from build123d import *

# Parameters (mm, degrees)
SKETCH1_R               = 225
BOSS_EXTRUDE1_DEPTH     = 30
SKETCH2_R               = 210
CUT_EXTRUDE1_DEPTH      = 1
CUT_EXTRUDE1_DEPTH_BACK = 31
SKETCH3_W               = 50
SKETCH3_H               = 20
BOSS_EXTRUDE2_DEPTH     = 50
SKETCH4_W               = 50
SKETCH4_H               = 20.506281323
BOSS_EXTRUDE3_DEPTH     = 110
SKETCH5_W               = 50
SKETCH5_H               = 25
BOSS_EXTRUDE7_DEPTH     = 40
SKETCH6_W               = 27.39243627
SKETCH6_H               = 13.13
BOSS_EXTRUDE8_DEPTH     = 15
SKETCH7_R               = 1.25
BOSS_EXTRUDE9_DEPTH     = 10
SKETCH8_R               = 1.25
BOSS_EXTRUDE10_DEPTH    = 10
FILLET14_R              = 3
FILLET15_R              = 2.5
FILLET17_R              = 3


with BuildPart() as part:
    # Sketch1 → Boss-Extrude1 (new body)
    with BuildSketch(Plane(origin=(0, 0, 0), x_dir=(1, 0, 0), z_dir=(0, 1, 0))):
        Circle(SKETCH1_R)
    extrude(amount=BOSS_EXTRUDE1_DEPTH)

    # Sketch2 → Cut-Extrude1 (cut, two sides)
    with BuildSketch(Plane(origin=(0, 30, 0), x_dir=(1, 0, 0), z_dir=(0, 1, 0))) as cut_extrude1_sk:
        Circle(SKETCH2_R)
    extrude(amount=CUT_EXTRUDE1_DEPTH, mode=Mode.SUBTRACT)
    extrude(cut_extrude1_sk.sketch, amount=-CUT_EXTRUDE1_DEPTH_BACK, mode=Mode.SUBTRACT)

    # Sketch3 → Boss-Extrude2 (add)
    with BuildSketch(Plane.XY.offset(-214.619360396)):
        with Locations((0, 15)):
            Rectangle(SKETCH3_W, SKETCH3_H)
    extrude(amount=-BOSS_EXTRUDE2_DEPTH)

    # Sketch4 → Boss-Extrude3 (add)
    with BuildSketch(Plane(origin=(0, 25, 0), x_dir=(1, 0, 0), z_dir=(0, 1, 0))):
        with Locations((0, 254.366219735)):
            Rectangle(SKETCH4_W, SKETCH4_H)
    extrude(amount=BOSS_EXTRUDE3_DEPTH)

    # Sketch5 → Boss-Extrude7 (add)
    with BuildSketch(Plane.XY.offset(-244.113079073)):
        with Locations((0, 122.5)):
            Rectangle(SKETCH5_W, SKETCH5_H)
    extrude(amount=BOSS_EXTRUDE7_DEPTH)

    # Sketch6 → Boss-Extrude8 (add)
    with BuildSketch(Plane.XY.offset(-204.113079073)):
        with Locations((0, 122.5)):
            Rectangle(SKETCH6_W, SKETCH6_H)
    extrude(amount=BOSS_EXTRUDE8_DEPTH)

    # Sketch7 → Boss-Extrude9 (add)
    with BuildSketch(Plane.ZY.offset(13.696218135)):
        with Locations((-196.613079073, 122.5)):
            Circle(SKETCH7_R)
    extrude(amount=BOSS_EXTRUDE9_DEPTH)

    # Sketch8 → Boss-Extrude10 (add)
    with BuildSketch(Plane(origin=(13.696218135, 0, 0), x_dir=(0, 0, -1), z_dir=(1, 0, 0))):
        with Locations((196.613079073, 122.5)):
            Circle(SKETCH8_R)
    extrude(amount=BOSS_EXTRUDE10_DEPTH)

    # Fillet14
    fillet14_edges = [part.edges().sort_by_distance(p)[0] for p in [
        (-13.696218135, 122.5, -189.113079073),
        (0, 115.935, -189.113079073),
        (13.696218135, 122.5, -189.113079073),
        (0, 129.065, -189.113079073),
    ]]
    fillet(fillet14_edges, radius=FILLET14_R)

    # Fillet15
    fillet15_edges = [part.edges().sort_by_distance(p)[0] for p in [
        (-13.696218135, 122.5, -204.113079073),
        (0, 115.935, -204.113079073),
        (13.696218135, 122.5, -204.113079073),
        (0, 129.065, -204.113079073),
        (-13.696218135, 122.5, -197.863079073),
        (13.696218135, 122.5, -195.363079073),
    ]]
    fillet(fillet15_edges, radius=FILLET15_R)

    # Fillet17
    fillet17_edges = [part.edges().sort_by_distance(p)[0] for p in [
        (0, 25, -225),
        (-25, 15, -223.60679775),
        (0, 5, -225),
        (25, 15, -223.60679775),
        (0, 5, -264.619360396),
        (0, 25, -244.113079073),
        (0, 135, -264.619360396),
        (0, 110, -204.113079073),
        (0, 135, -204.113079073),
    ]]
    fillet(fillet17_edges, radius=FILLET17_R)


solid = part.part
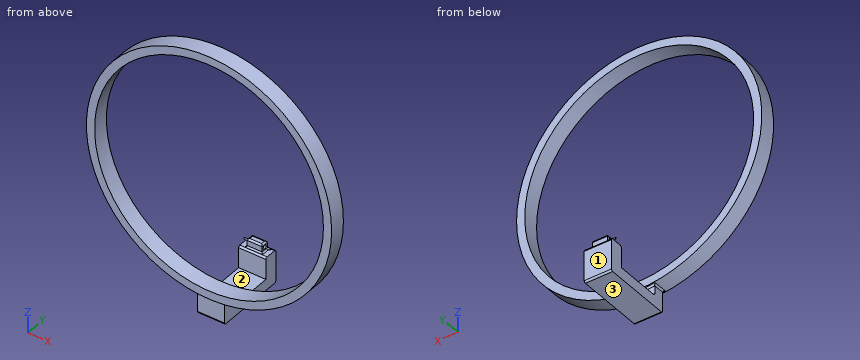
The model under review builds one solid part; all positions refer to its coordinate system, in mm. Face numbers are marked on the shaded views. Give positions to 0.01 mm unless a question says otherwise; leave off trailing zeros. Order: outer loops, then holes, each group sorted by start corner. A loop starts at its lowest first (then second) coordinate and runs counter-clockwise, first axis right, second up. Notation, with made-up numbers: M 65.25,53.5 L 109.25,53.5 A7 ccw 109.25,64.5 Z; hole C 58.25,-17 d11. An arc over 180 degrees is marked long. Answer in a Markdown table with one row per item. Add a question column.
1. Add section B-B on y = 18. State the section outline as (x, z) points.
2. Add section C-C on z = 77. State the section outline as (x, y) points.
3. Add section D-D on x = -53. State the section outline as (y, z) points.
4. Mouldability with a two-part tool opening along Y and no side actions: class the marked faces 1, 2 and 3 as released by +Y, released by -Y, zero draft, split by the parting line, or undercut.
5. For pin 1 Ø4 at (y, z) = (29, -148.5) entering from +X; pin 2 Ø5 at (y, z) = (124, -195) entering from -X; pin 3 Ø5.5 at (x, y) = (0.5, 120) entering from +Z, all flat-tipped, find the tip position at first contact; note any pin that passes through.
6. To check wall thickness, follow line 1 along X through (y, z) = (6, 0); line 2 along Z through (x, y) = (0, 17); line 3 along Y through (x, z) = (179, -135.5). State the ranges of each line that lie inside material, in increasing order.
The answers:
| question | item | result |
|---|---|---|
| 1 | outline | M -27.63,-223.3 A3 cw -25,-226.27 L -25,-264.62 L 25,-264.62 L 25,-226.27 A3 cw 27.63,-223.3 A225 ccw long Z; hole C 0,0 d420 |
| 2 | outline | M -211.41,0 L -195.37,0 L -195.37,30 L -211.41,30 Z; M 195.37,0 L 211.41,0 L 211.41,30 L 195.37,30 Z |
| 3 | outline | M 0,-218.67 L 30,-218.67 L 30,-203.2 L 0,-203.2 Z; M 0,203.2 L 30,203.2 L 30,218.67 L 0,218.67 Z |
| 4 | face 1 | released by +Y |
| 4 | face 2 | undercut |
| 4 | face 3 | zero draft |
| 5 | pin 1 | x = 170.77 |
| 5 | pin 2 | x = -23.7 |
| 5 | pin 3 | z = -189.11 |
| 6 | line 1 | -225 to -210, 210 to 225 |
| 6 | line 2 | -264.62 to -210, 210 to 225 |
| 6 | line 3 | 0 to 30 |
